CAD build for the part. Positions are in the model's coordinates, mm. A direction names the side the tool comes from. Coordinates: 2 decimals unless noted, no trailing zeros. Write each loop counter-clockwise with the first axis right and the second up, starting at its lowest first coordinate (ties: lowest second). Pieces come first, ordered by that corner, then holes. Notation, with made-up numbers: (18, 28) - (38, 28) arc R4 cw to (38, 35) - close; hole circle Ø8 at (49, -15). An arc over 180 degrees is marked (long way). One line per question, with ' | ' between items. Start each with the question number.
1. Probe line 1 (Z direction, x = -3.5, y = 6.25) (3 decimals); line 2 (X direction, y = 7, z = 2.75); line 3 (X direction, y = 3.25, z = 4.5). List the from-to ranges inside material, lowest first.
2. Band-saw the part on A-A, the plane y = 8.25. Write the cut outline in (x, z) (3 decimals).
3. Which spindle directions (+Z, -Z, +X, -X, +Y, -Y) get a long thin tool onto all of the face, cutting with end or side? Do faces 5 (the flat face through (-13, 6, 0.75)), 6 (the cylindrical face through (-25.859, 9.297, 3.422)). Say none if no direction does.
4. Band-saw the part on C-C, the plane x = -3.5. Write the cut outline in (y, z) (3 decimals), then the cut area to 3 significant figures.
5. Band-saw the part on D-D, the plane y = 5. Write the cut outline in (x, z) (3 decimals).
6. Two-plate mould, pull along X, no slides. Class faces 1 (the flat face through (0, 3, 3)), 2 (the cylindrical face through (-13.4, 4.5, 0.4)), 3 (the flat face through (-27, 3, 3)), 4 (the flat face through (-6, 10.5, 3)): +X half, -X half, draft (parallel to the pull), parting line (faces both ways), or undercut.
7. Band-saw the part on B-B, the plane z = 4. Write the cut outline in (x, y).
from build123d import *

# Parameters (mm, degrees)
BOSS_EXTRUDE1_DEPTH = 6.75
SKETCH3_R           = 8
CUT_EXTRUDE2_DEPTH  = 0.75
SKETCH4_W           = 27
SKETCH4_H           = 2
CUT_EXTRUDE3_DEPTH  = 9
SKETCH5_R           = 1.5
CUT_EXTRUDE4_DEPTH  = 16
FILLET1_R           = 4


with BuildPart() as part:
    # Sketch1 → Boss-Extrude1 (new body)
    with BuildSketch(Plane.XY):
        with BuildLine():
            Line((-27, 0), (0, 0))
            Line((0, 0), (0, 12.5))
            Line((0, 12.5), (-7.5, 12.5))
            ThreePointArc((-7.5, 12.5), (-13.5, 6.5), (-19.5, 12.5))
            Line((-19.5, 12.5), (-27, 12.5))
            Line((-27, 12.5), (-27, 0))
        make_face()
    extrude(amount=BOSS_EXTRUDE1_DEPTH)

    # Sketch3 → Cut-Extrude2 (cut)
    with BuildSketch(Plane(origin=(0, 0, 0), x_dir=(-1, 0, 0), z_dir=(0, 0, -1))):
        with Locations((13.5, 12.5)):
            Circle(SKETCH3_R)
    extrude(amount=-CUT_EXTRUDE2_DEPTH, mode=Mode.SUBTRACT)

    # Sketch4 → Cut-Extrude3 (cut)
    with BuildSketch(Plane.XY.offset(6.75)):
        with Locations((-13.5, 11.5)):
            Rectangle(SKETCH4_W, SKETCH4_H)
    extrude(amount=-CUT_EXTRUDE3_DEPTH, mode=Mode.SUBTRACT)

    # Sketch5 → Cut-Extrude4 (cut)
    with BuildSketch(Plane.XZ):
        with Locations((-23.5, 3.375)):
            Circle(SKETCH5_R)
        with Locations((-3.5, 3.375)):
            Circle(SKETCH5_R)
    extrude(amount=-CUT_EXTRUDE4_DEPTH, mode=Mode.SUBTRACT)

    # Fillet1
    # the kernel refuses this fillet: 4 mm, written as the material it takes off along each edge
    with BuildSketch(Plane(origin=(-27, 10.5, 16.75), x_dir=(1, 0, 0), z_dir=(0, 0, -1))) as fillet1_piece_1:
        with BuildLine():
            CenterArc((FILLET1_R, FILLET1_R), FILLET1_R, 180, 90)
            Line((0, FILLET1_R), (0, 0))
            Line((0, 0), (FILLET1_R, 0))
        make_face()
    extrude(amount=26.75, mode=Mode.SUBTRACT)
    with BuildSketch(Plane(origin=(0, 10.5, 16.75), x_dir=(-1, 0, 0), z_dir=(0, 0, -1))) as fillet1_piece_2:
        with BuildLine():
            CenterArc((FILLET1_R, -FILLET1_R), FILLET1_R, 90, 90)
            Line((0, -FILLET1_R), (0, 0))
            Line((0, 0), (FILLET1_R, 0))
        make_face()
    extrude(amount=26.75, mode=Mode.SUBTRACT)


solid = part.part
Filled in:
1) line 1: z = 0 to 1.875, 4.875 to 6.75 | line 2: x = -26.97 to -24.86, -22.14 to -15.9, -11.1 to -4.86, -2.14 to -0.03 | line 3: x = -27 to -24.49, -22.51 to -4.49, -2.51 to 0
2) outline: (-26.597, 0) - (-20.278, 0) - (-20.278, 0.75) - (-17.735, 0.75) - (-17.735, 6.75) - (-26.597, 6.75) - close; (-9.265, 0.75) - (-6.722, 0.75) - (-6.722, 0) - (-0.403, 0) - (-0.403, 6.75) - (-9.265, 6.75) - close; hole circle Ø3 at (-23.5, 3.375); hole circle Ø3 at (-3.5, 3.375)
3) face 5: -Z, +Y | face 6: +Z, -Z, -X, +Y
4) outline: (0, 0) - (10.469, 0) - (10.469, 1.875) - (0, 1.875) - close; (0, 4.875) - (10.469, 4.875) - (10.469, 6.75) - (0, 6.75) - close | area: 39.3 mm²
5) outline: (-27, 0) - (-16.284, 0) - (-16.284, 0.75) - (-10.716, 0.75) - (-10.716, 0) - (0, 0) - (0, 6.75) - (-27, 6.75) - close; hole circle Ø3 at (-23.5, 3.375); hole circle Ø3 at (-3.5, 3.375)
6) face 1: +X half | face 2: undercut | face 3: -X half | face 4: draft
7) outline: (-27, 0) - (-24.86, 0) - (-24.86, 10.04) arc R4 ccw to (-27, 6.5) - close; (-22.14, 0) - (-4.86, 0) - (-4.86, 10.5) - (-7.84, 10.5) arc R6 cw to (-19.16, 10.5) - (-22.14, 10.5) - close; (-2.14, 0) - (0, 0) - (0, 6.5) arc R4 ccw to (-2.14, 10.04) - close
